from build123d import *

# Parameters (mm, degrees)
ESQUISSE2_W             = 200
ESQUISSE2_H             = 80
BOSS_EXTRU_1_DEPTH      = 3.175
ESQUISSE3_W             = 35
ESQUISSE3_H             = 3.175
ENL_V_MAT_EXTRU_1_DEPTH = 4.175
ESQUISSE4_W             = 3.175
ESQUISSE4_H             = 22.5
ENL_V_MAT_EXTRU_2_DEPTH = 4.175


with BuildPart() as part:
    # Esquisse2 → Boss.-Extru.1 (new body)
    with BuildSketch(Plane.XY):
        Rectangle(ESQUISSE2_W, ESQUISSE2_H)
    extrude(amount=BOSS_EXTRU_1_DEPTH)

    # Esquisse3 → Enlèv. mat.-Extru.1 (cut, through all)
    with BuildSketch(Plane.XY.offset(3.175)):
        with Locations((35, 38.4125)):
            Rectangle(ESQUISSE3_W, ESQUISSE3_H)
        with Locations((-35, 38.4125)):
            Rectangle(ESQUISSE3_W, ESQUISSE3_H)
    extrude(amount=-ENL_V_MAT_EXTRU_1_DEPTH, mode=Mode.SUBTRACT)

    # Esquisse4 → Enlèv. mat.-Extru.2 (cut, through all)
    with BuildSketch(Plane.XY.offset(3.175)):
        with Locations((-98.4125, 28.75)):
            Rectangle(ESQUISSE4_W, ESQUISSE4_H)
        with Locations((-98.4125, -28.75)):
            Rectangle(ESQUISSE4_W, ESQUISSE4_H)
    enl_v_mat_extru_2 = extrude(amount=-ENL_V_MAT_EXTRU_2_DEPTH, mode=Mode.SUBTRACT)

    # Symétrie1: Enlèv. mat.-Extru.2 across plane
    add(enl_v_mat_extru_2.mirror(Plane(origin=(0, 0, 0), x_dir=(0, 0, 1), z_dir=(1, 0, 0))), mode=Mode.SUBTRACT)


solid = part.part
The model under review builds one solid part; all positions refer to its coordinate system, in mm. Coordinates: 2 decimals unless noted, no trailing zeros. Write each loop counter-clockwise with the first axis right and the second up, starting at its lowest first coordinate (ties: lowest second). Pieces come first, ordered by that corner, then holes. Notation, with made-up numbers: M -18,0 L -4,0 A21 cw -4,15 Z; hole C -30.75,85 d11. An arc over 180 degrees is marked long. Put each result on its own line as item: value.
1) Add section A-A on z = 1.2. Give the boundary of the cut face in (x, y) (3 decimals), then the cut area to 3 significant figures.
Computed:
outline: M -100,-17.5 L -96.825,-17.5 L -96.825,-40 L 96.825,-40 L 96.825,-17.5 L 100,-17.5 L 100,17.5 L 96.825,17.5 L 96.825,40 L 52.5,40 L 52.5,36.825 L 17.5,36.825 L 17.5,40 L -17.5,40 L -17.5,36.825 L -52.5,36.825 L -52.5,40 L -96.825,40 L -96.825,17.5 L -100,17.5 Z
area: 15,500 mm2
2) Wall thickness on probe 1 along Y at (x, z) = (20.5, 2.9) (3 decimals); probe 2 along X at (y, z) = (28.5, 1.8) (3 decimals): over which ranges is each line inside the solid? List them lowest first. Write a range as [from, to].
Computed:
probe 1: y = [-40, 36.825]
probe 2: x = [-96.825, 96.825]
3) Add section C-C on y = 34.5. Give the boundary of the cut face in (x, z) (3 decimals), then the cut area to 3 significant figures.
Computed:
outline: M -96.825,0 L 96.825,0 L 96.825,3.175 L -96.825,3.175 Z
area: 615 mm2
4) Clearance check with flat-ended pins moving along their axes: pin 1 Ø1.6 at (y, z) = (38.5, 1) entering from +X (3 decimals); pin 2 Ø1.6 at (y, z) = (39, 1) entering from -X (3 decimals); pin 3 Ø2 at (x, y) = (-25.5, 18) entering from -Z; pin 4 Ø1.6 at (x, z) = (27.5, 1) entering from +Y (3 decimals). State where each tip first meets the part, or that it passes through.
Computed:
pin 1: stops at x = 96.825
pin 2: stops at x = -96.825
pin 3: stops at z = 0
pin 4: stops at y = 36.825
5) Add section B-B on x = -29.5. Give the boundary of the cut face in (y, z) (3 decimals).
Computed:
outline: M -40,0 L 36.825,0 L 36.825,3.175 L -40,3.175 Z
